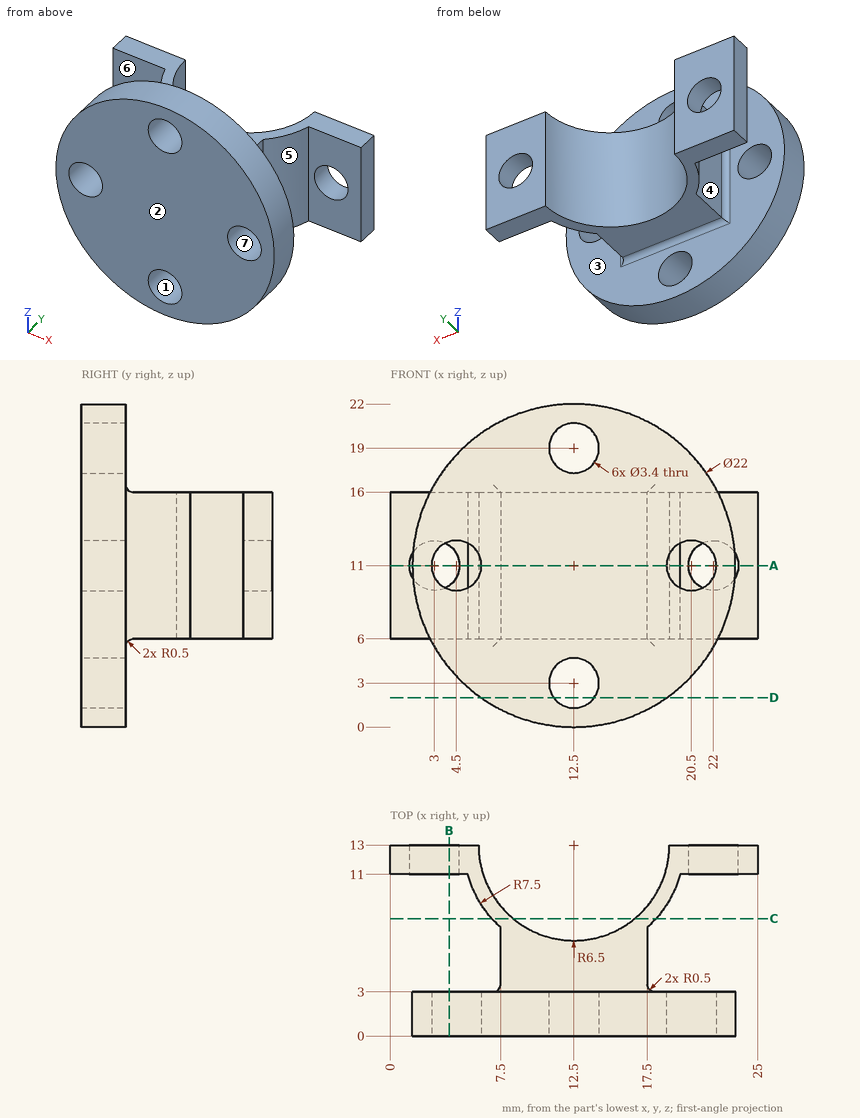
Geometry check sheet. Reference: drawing and pictorial views, mm from the part's lowest x, y, z. A direction names the side the tool comes from. Coordinates: 2 decimals unless noted, no trailing zeros. Order: outer loops, then holes, each group sorted by start corner. A loop starts at its lowest first (then second) coordinate and runs counter-clockwise, first axis right, second up.
1. Scan lines: line 1 (Y direction, x = 5, z = 7.75); line 2 (Z direction, x = 3, y = 12); line 3 (Z direction, x = 11, y = 1). Record each from-to range of solid material in increasing order.
Results found:
line 1: y = 0 to 3, 11 to 13
line 2: z = 6 to 9.3, 12.7 to 16
line 3: z = 0.1 to 2.2, 3.8 to 18.2, 19.8 to 21.9
2. Sectioned sample at B-B, the plane x = 4. Record the cut outline in (y, z), and give its area (3 significant figures).
Results found:
outline: (0, 4.02) - (3, 4.02) - (3, 9.38) - (0, 9.38) - close; (0, 12.62) - (3, 12.62) - (3, 17.98) - (0, 17.98) - close; (11, 6) - (13, 6) - (13, 9.63) - (11, 9.63) - close; (11, 12.37) - (13, 12.37) - (13, 16) - (11, 16) - close
area: 46.6 mm2
3. Sectioned sample at C-C, the plane y = 8. Record the cut outline in (x, z).
Results found:
outline: (6.91, 6) - (8.35, 6) - (8.35, 16) - (6.91, 16) - close; (16.65, 6) - (18.09, 6) - (18.09, 16) - (16.65, 16) - close
4. Release check for a two-part mould opening along Y. For the marked faces 1, 2, 3 and 4 record: +Y half, -Y half, draft (parallel to the pull), parting line (faces both ways), or undercut.
Results found:
face 1: draft
face 2: -Y half
face 3: undercut
face 4: undercut
5. Set-up check for the marked faces 5, 6 and 7: record each of +Z, -Z, +X, -X, +Y, -Y from which the full face is reachable in a straight line by a thin tool's end or side.
Results found:
face 5: +Z, -Z, +X
face 6: +Z, -Z, -X
face 7: -Y
6. Sectioned sample at A-A, the plane z = 11. Give the number of separate pieces and of enclosed holes in the cut face, and give its area (3 significant figures).
Results found:
separate pieces: 5
enclosed holes: 0
area: 105 mm2
7. Sectioned sample at D-D, the plane z = 2. Record the cut outline in (x, y).
Results found:
outline: (6.18, 0) - (11.13, 0) - (11.13, 3) - (6.18, 3) - close; (13.87, 0) - (18.82, 0) - (18.82, 3) - (13.87, 3) - close
8. Go/stop test with flat-tipped pins: pin 1 Ø4 at (x, z) = (12.5, 19) entering from +Y; pin 2 Ø3 at (y, z) = (5.5, 10.5) entering from -X; pin 3 Ø2 at (y, z) = (6, 9) entering from +X. Record where each tip stops, or that it passes through.
Results found:
pin 1: stops at y = 3
pin 2: stops at x = 7.5
pin 3: stops at x = 17.5
